```python
from build123d import *

# Parameters (mm, degrees)
SKETCH_1_W                = 80
SKETCH_1_H                = 40
EXTRUDE_228_DEPTH         = 6
CUT_EXTRUDE_M4_DEPTH      = 46.122056691
CUT_EXTRUDE_M4_DEPTH_BACK = 46.122056691
SKETCH_2_R                = 2.25


with BuildPart() as part:
    # 草图1 → Extrude 228 (new body)
    with BuildSketch(Plane.XY):
        Rectangle(SKETCH_1_W, SKETCH_1_H)
    extrude(amount=EXTRUDE_228_DEPTH)

    # 草图2 → 拼接M4孔 (cut, two sides: drawn at the far end of the back side and taken through both)
    with BuildSketch(Plane.XY.offset(-CUT_EXTRUDE_M4_DEPTH_BACK)):
        with Locations((-25, -10)):
            Circle(SKETCH_2_R)
        with Locations((-25, 10)):
            Circle(SKETCH_2_R)
        with Locations((25, -10)):
            Circle(SKETCH_2_R)
        with Locations((25, 10)):
            Circle(SKETCH_2_R)
    extrude(amount=CUT_EXTRUDE_M4_DEPTH + CUT_EXTRUDE_M4_DEPTH_BACK, mode=Mode.SUBTRACT)


solid = part.part
```
The model under review builds one solid part; all positions refer to its coordinate system, in mm. Give positions to 0.01 mm unless a question says otherwise; leave off trailing zeros. Write each loop counter-clockwise with the first axis right and the second up, starting at its lowest first coordinate (ties: lowest second). Pieces come first, ordered by that corner, then holes. Notation, with made-up numbers: M -21.5,42.25 L 5.5,42.25 A18 cw 5.5,63.25 Z; hole C -34,58 d6. An arc over 180 degrees is marked long. Answer in a Markdown table with one row per item.
Item 1: For line 1 along Y through (x, z) = (-25, 1.3); line 2 along X through (y, z) = (-10, 2); line 3 along X through (y, z) = (-8, 1.7), list the stretches that pass through material, from the lowest coordinate up.
Check sheet entries:
| item | result |
|---|---|
| line 1 | -20 to -12.25, -7.75 to 7.75, 12.25 to 20 |
| line 2 | -40 to -27.25, -22.75 to 22.75, 27.25 to 40 |
| line 3 | -40 to -26.03, -23.97 to 23.97, 26.03 to 40 |
Item 2: Add section A-A on z = 4.45. Give the boundary of the cut face in (x, y), plus the area to 3 significant figures.
Check sheet entries:
| item | result |
|---|---|
| outline | M -40,-20 L 40,-20 L 40,20 L -40,20 Z; hole C -25,-10 d4.5; hole C -25,10 d4.5; hole C 25,-10 d4.5; hole C 25,10 d4.5 |
| area | 3,140 mm2 |
Item 3: Add section B-B on x = 25. Give the boundary of the cut face in (y, z).
Check sheet entries:
| item | result |
|---|---|
| outline | M -20,0 L -12.25,0 L -12.25,6 L -20,6 Z; M -7.75,0 L 7.75,0 L 7.75,6 L -7.75,6 Z; M 12.25,0 L 20,0 L 20,6 L 12.25,6 Z |
Item 4: Add section C-C on y = -10. Give the boundary of the cut face in (x, z), plus the area to 3 significant figures.
Check sheet entries:
| item | result |
|---|---|
| outline | M -40,0 L -27.25,0 L -27.25,6 L -40,6 Z; M -22.75,0 L 22.75,0 L 22.75,6 L -22.75,6 Z; M 27.25,0 L 40,0 L 40,6 L 27.25,6 Z |
| area | 426 mm2 |
Item 5: Draft analysis for pull direction Y (two halves, no side actions). For faces 1 (the face through (26.21, -8.103, 2.958)), 2 (the face through (-1, 20, 3)), 3 (the face through (-1, 0, 6)), state which applies: +Y half, -Y half, draft (parallel to the pull), parting line (faces both ways), or undercut.
Check sheet entries:
| item | result |
|---|---|
| face 1 | undercut |
| face 2 | +Y half |
| face 3 | draft |
